Read the model definition and answer for the solid it produces. Units are mm, in the model's axes. A direction names the side the tool comes from. Coordinates: 2 decimals unless noted, no trailing zeros. Write each loop counter-clockwise with the first axis right and the second up, starting at its lowest first coordinate (ties: lowest second). Pieces come first, ordered by that corner, then holes. Notation, with made-up numbers: (12, 66) -> (18, 66) arc R24 cw to (18, 94) -> close; hole circle Ø11 at (66, 54.25). An arc over 180 degrees is marked (long way). Write item = value, one per line. Start each with the question number.
1) Section D-D (y = 139.5) is taken. Determine the outline of the cut face in (x, z), plus the area to 3 significant figures.
2) A flat-ended cylindrical pin translates along its axis: pin 1 Ø6 at (x, y) = (166.42, 231.17) entering from +Z. Find the tip coordinate at first contact, or state that the pin passes through.
3) Section C-C (y = 170.5) is taken. Determine the outline of the cut face in (x, z), plus the area to 3 significant figures.
4) For a pull along X with two mould halves and no side action, classify faces 3 (the face through (410.023, 117.579, 4.479)), 4 (the face through (146, 229, 6)) as released by +X, released by -X, zero draft, split by the parting line, or undercut.
5) A tool of negligible diameter and unlimited length cuts with its end or side. For faces 1 (the face through (-77.18, 214.766, 4.479)), 2 (the face through (170, 167, 0)), from which of +Z, -Z, +X, -X, +Y, -Y can it reach the whole face along a straight path? Write none if from no direction.
6) Find the intervals of material crossed by line 1 along Y through (x, z) = (103, 5); line 2 along X through (y, z) = (147.5, 3.5); line 3 along Z through (x, y) = (58.5, 132), in increasing order. Write a range as from..to.
7) Section A-A (x = 357) is taken. Determine the outline of the cut face in (y, z), plus the area to 3 significant figures.
8) Section B-B (z = 4.2) is taken. Determine the outline of the cut face in (x, y).
from build123d import *

# Parameters (mm, degrees)
AUFSATZ_LINEAR_AUSTRAGEN1_DEPTH = 3
SKIZZE2_W                       = 52.543234094
SKIZZE2_H                       = 140
SKIZZE2_W_2                     = 111.276179835
AUFSATZ_LINEAR_AUSTRAGEN2_DEPTH = 3
VERRUNDUNG1_R                   = 50
VERRUNDUNG2_R                   = 50
SKIZZE3_R                       = 2.5
SCHNITT_LINEAR_AUSTRAGEN1_DEPTH = 10
AUFSATZ_LINEAR_AUSTRAGEN3_DEPTH = 3
SKIZZE6_R                       = 2.5
SCHNITT_LINEAR_AUSTRAGEN2_DEPTH = 7


with BuildPart() as part:
    # Skizze1 → Aufsatz-Linear austragen1 (new body)
    with BuildSketch(Plane.XY):
        Polygon((432.051221513, 126.172344807), (432.051221513, 206.172344807), (431.494421695, 212.025054468), (429.845419749, 217.652847778), (427.167585893, 222.839451798), (423.563827781, 227.385548243), (419.172635816, 231.116433176), (414.162761042, 233.888730783), (408.726730139, 235.595903219), (403.073446724, 236.172344807), (-70.230208158, 236.172344807), (-75.883491573, 235.595903219), (-81.319522476, 233.888730783), (-86.32939725, 231.116433176), (-90.720589215, 227.385548243), (-94.324347327, 222.839451798), (-97.002181183, 217.652847778), (-98.651183129, 212.025054468), (-99.207982946, 206.172344807), (-99.207982946, 126.172344807), (-98.651183129, 120.319635147), (-97.002181183, 114.691841836), (-94.324347327, 109.505237817), (-90.720589215, 104.959141372), (-86.32939725, 101.228256438), (-81.319522476, 98.455958832), (-75.883491573, 96.748786395), (-70.230208158, 96.172344807), (403.073446724, 96.172344807), (408.726730139, 96.748786395), (414.162761042, 98.455958832), (419.172635816, 101.228256438), (423.563827781, 104.959141372), (427.167585893, 109.505237817), (429.845419749, 114.691841836), (431.494421695, 120.319635147), align=None)
    extrude(amount=AUFSATZ_LINEAR_AUSTRAGEN1_DEPTH)

    # Skizze2 → Aufsatz-Linear austragen2 (add)
    with BuildSketch(Plane(origin=(0, 0, 0), x_dir=(-1, 0, 0), z_dir=(0, 0, -1))):
        with Locations((-405.779604466, 166.172344807)):
            Rectangle(SKIZZE2_W, SKIZZE2_H)
        with Locations((43.569893028, 166.172344807)):
            Rectangle(SKIZZE2_W_2, SKIZZE2_H)
    extrude(amount=-AUFSATZ_LINEAR_AUSTRAGEN2_DEPTH)

    # Verrundung1
    verrundung1_edges = [part.edges().sort_by_distance(p)[0] for p in [
        (432.051221513, 96.172344807, 1.5),
        (-99.207982946, 236.172344807, 1.5),
        (-99.207982946, 96.172344807, 1.5),
    ]]
    fillet(verrundung1_edges, radius=VERRUNDUNG1_R)

    # Verrundung2
    verrundung2_edges = [part.edges().sort_by_distance(p)[0] for p in [
        (432.051221513, 236.172344807, 1.5),
    ]]
    fillet(verrundung2_edges, radius=VERRUNDUNG2_R)

    # Skizze3 → Schnitt-Linear austragen1 (cut)
    with BuildSketch(Plane.XY.offset(3)):
        with Locations((166.421619283, 231.172344807)):
            Circle(SKIZZE3_R)
    extrude(amount=-SCHNITT_LINEAR_AUSTRAGEN1_DEPTH, mode=Mode.SUBTRACT)

    # Skizze5 → Aufsatz-Linear austragen3 (add)
    with BuildSketch(Plane.XY.offset(3)):
        with BuildLine():
            Line((432.051221513, 146.172344807), (432.051221513, 186.172344807))
            ThreePointArc((432.051221513, 186.172344807), (417.406560572, 221.527683867), (382.051221513, 236.172344807))
            Line((382.051221513, 236.172344807), (-49.207982946, 236.172344807))
            ThreePointArc((-49.207982946, 236.172344807), (-84.563322006, 221.527683867), (-99.207982946, 186.172344807))
            Line((-99.207982946, 186.172344807), (-99.207982946, 146.172344807))
            ThreePointArc((-99.207982946, 146.172344807), (-84.563322006, 110.817005748), (-49.207982946, 96.172344807))
            Line((-49.207982946, 96.172344807), (382.051221513, 96.172344807))
            ThreePointArc((382.051221513, 96.172344807), (417.406560572, 110.817005748), (432.051221513, 146.172344807))
        make_face()
        with BuildLine():
            Line((-89.207982946, 186.172344807), (-89.207982946, 146.172344807))
            ThreePointArc((-89.207982946, 146.172344807), (-77.492254194, 117.88807356), (-49.207982946, 106.172344807))
            Line((-49.207982946, 106.172344807), (382.051221513, 106.172344807))
            ThreePointArc((382.051221513, 106.172344807), (410.33549276, 117.88807356), (422.051221513, 146.172344807))
            Line((422.051221513, 146.172344807), (422.051221513, 186.172344807))
            ThreePointArc((422.051221513, 186.172344807), (410.33549276, 214.456616055), (382.051221513, 226.172344807))
            Line((382.051221513, 226.172344807), (-49.207982946, 226.172344807))
            ThreePointArc((-49.207982946, 226.172344807), (-77.492254194, 214.456616055), (-89.207982946, 186.172344807))
        make_face(mode=Mode.SUBTRACT)
    extrude(amount=AUFSATZ_LINEAR_AUSTRAGEN3_DEPTH)

    # Skizze6 → Schnitt-Linear austragen2 (cut, through all)
    with BuildSketch(Plane(origin=(0, 0, 0), x_dir=(-1, 0, 0), z_dir=(0, 0, -1))):
        with Locations(Location((-166.421619283, 231.172344807, 0), (0, 0, 180))):  # turned: the seam where the file's is
            Circle(SKIZZE6_R)
    extrude(amount=-SCHNITT_LINEAR_AUSTRAGEN2_DEPTH, mode=Mode.SUBTRACT)


solid = part.part
Answer key:
q1.outline = (-98.76, 0) -> (431.6, 0) -> (431.6, 6) -> (421.49, 6) -> (421.49, 3) -> (-88.65, 3) -> (-88.65, 6) -> (-98.76, 6) -> close
q1.area = 1,650 mm^2
q2.pin_1 = 6
q3.outline = (-99.21, 0) -> (432.05, 0) -> (432.05, 6) -> (422.05, 6) -> (422.05, 3) -> (-89.21, 3) -> (-89.21, 6) -> (-99.21, 6) -> close
q3.area = 1,650 mm^2
q4.face_3 = undercut
q4.face_4 = zero draft
q5.face_1 = +Z
q5.face_2 = -Z, +X, -X, +Y, -Y
q6.line_1 = 96.17..106.17, 226.17..236.17
q6.line_2 = -99.21..-89.21, 422.05..432.05
q6.line_3 = 0..3
q7.outline = (96.17, 0) -> (236.17, 0) -> (236.17, 6) -> (226.17, 6) -> (226.17, 3) -> (106.17, 3) -> (106.17, 6) -> (96.17, 6) -> close
q7.area = 480 mm^2
q8.outline = (-99.21, 146.17) arc R50 ccw to (-49.21, 96.17) -> (382.05, 96.17) arc R50 ccw to (432.05, 146.17) -> (432.05, 186.17) arc R50 ccw to (382.05, 236.17) -> (-49.21, 236.17) arc R50 ccw to (-99.21, 186.17) -> close; hole (-89.21, 146.17) arc R40 ccw to (-49.21, 106.17) -> (382.05, 106.17) arc R40 ccw to (422.05, 146.17) -> (422.05, 186.17) arc R40 ccw to (382.05, 226.17) -> (-49.21, 226.17) arc R40 ccw to (-89.21, 186.17) -> close; hole circle Ø5 at (166.42, 231.17)
